Can you work these out from the drawing? Everything is in mm from the part's minimum corner. A direction names the side the tool comes from. Give positions to 0.01 mm unless a question says otherwise; leave off trailing zeros. Order: outer loops, then holes, each group sorted by start corner. A loop starts at its lowest first (then second) coordinate and runs counter-clockwise, first axis right, second up. Notation, with made-up numbers: M 80.25,15.25 L 106.25,15.25 A26 ccw 106.25,54.25 Z; hole C 71.5,-1.75 d5. An arc over 180 degrees is marked long. Answer as a JSON object with one key per item and string values.
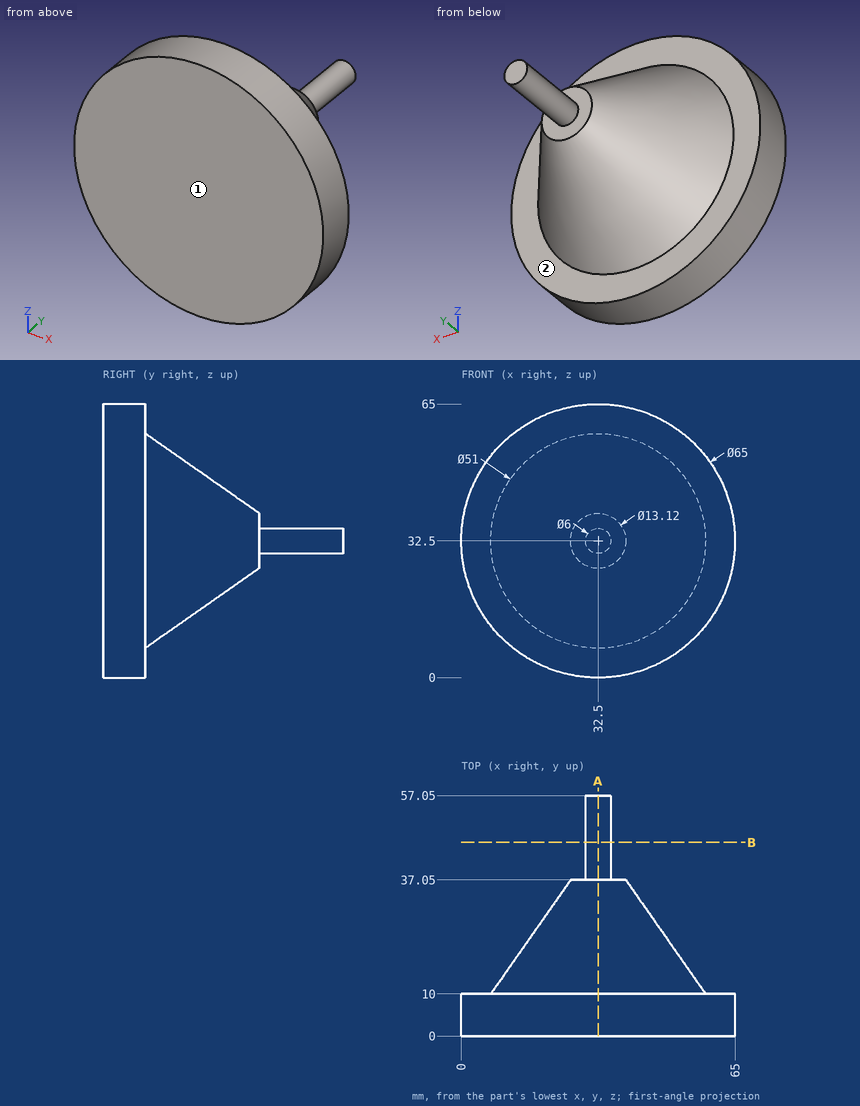
1) I need wall thicknesses on L1, parallel to Y at x = 61, z = 19.5; L2, parallel to X at y = 4, z = 17.5; L3, parallel to X at y = 26.5, z = 41. Which ranges of each line are inside material? Lowest first, please.
Results found:
{"L1": "y = 0 to 10", "L2": "x = 3.67 to 61.33", "L3": "x = 21.44 to 43.56"}
2) I'm going to push flat-ended pins straight in: pin 1 Ø1.5 at (x, y) = (31, 44.5) entering from -Z; pin 2 Ø10 at (x, z) = (14.5, 47) entering from -Y; pin 3 Ø4 at (y, z) = (22.5, 34.5) entering from +X; pin 4 Ø10 at (y, z) = (46, 43.5) entering from -X. Where does each tip first touch, or does it pass through?
Results found:
{"pin 1": "stops at z = 29.6", "pin 2": "stops at y = 0", "pin 3": "stops at x = 50.55", "pin 4": "passes through"}
3) I want a section at A-A on x = 32.5. Write out the boundary of the cut face in (y, z).
Results found:
{"outline": "M 0,0 L 10,0 L 10,7 L 37.05,25.94 L 37.05,29.5 L 57.05,29.5 L 57.05,35.5 L 37.05,35.5 L 37.05,39.06 L 10,58 L 10,65 L 0,65 Z"}
4) For the marked faces 1 and 2, which set-ups out of +Z, -Z, +X, -X, +Y, -Y let a thin tool reach every point of the face, with its end or its side?
Results found:
{"face 1": "+Z, -Z, +X, -X, -Y", "face 2": "+Y"}
5) I want a section at B-B on y = 46. Write out the boundary of the cut face in (x, z).
Results found:
{"outline": "C 32.5,32.5 d6"}
